Here's how the part is built. I have some questions about the finished solid (model axes, mm). Face numbers are marked on the shaded views. A direction names the side the tool comes from. Give positions to 0.01 mm unless a question says otherwise; leave off trailing zeros. Write each loop counter-clockwise with the first axis right and the second up, starting at its lowest first coordinate (ties: lowest second). Pieces come first, ordered by that corner, then holes. Notation, with made-up numbers: (59.5, 34.5) - (68.5, 34.5) arc R24 ccw to (68.5, 48.5) - close; hole circle Ø3 at (17, 10.5). An arc over 180 degrees is marked (long way). Write each question's results on one line, items separated by ' | '. Start each with the question number.
Item 1: Suppose I cut it at B-B on z = 0. List the corners of the cut face in (x, y) for me.
Item 2: Please list where these lines run through material, in increasing order: line 1 along X through (y, z) = (-3.75, 0); line 2 along Y through (x, z) = (14.5, 9.5); line 3 along Z through (x, y) = (-2.5, 0.75).
Item 3: Suppose I cut it at C-C on y = 1. List the corners of the cut face in (x, z) for me, then the cut area to 3 significant figures.
Item 4: We'd pull the mould along X, two halves only. Please class the marked faces 1, 2 and 3: +X half, -X half, draft (parallel to the pull), parting line (faces both ways), or undercut.
Item 5: Will these pins go through, and if not, where does the flat tip stop? P1, Ø1.5, axis at y = 5, z = 21, coming from the +X side; P2, Ø2, axis at x = -17, z = 15.5, coming from the -Y side; P3, Ø6, axis at y = 1, z = -18, coming from the +X side; P4, Ø8, axis at x = 0, z = 0, coming from the +Y side.
Item 6: Which directions (+Z, -Z, +X, -X, +Y, -Y) give clear straight access to the entire face, cutting with the end or side of a thin tool? Please do the marked faces 4 and 5.
Item 7: Suppose I cut it at A-A on x = 0. List the corners of the cut face in (y, z) for me.
```python
from build123d import *


with BuildPart() as part:
    # Sketch → Revolution (revolve)
    with BuildSketch(Plane.YZ):
        Polygon((7, 40), (-7, 40), (-4.57259, 33.620199), (-4.57259, 9.331906), (-7, 9.331906), (-7, 5), (7, 5), (7, 9.331906), (4.57259, 9.331906), (4.57259, 33.620199), align=None)
    revolve(axis=Axis((0, 0, 0), (0, 1, 0)))


solid = part.part
```
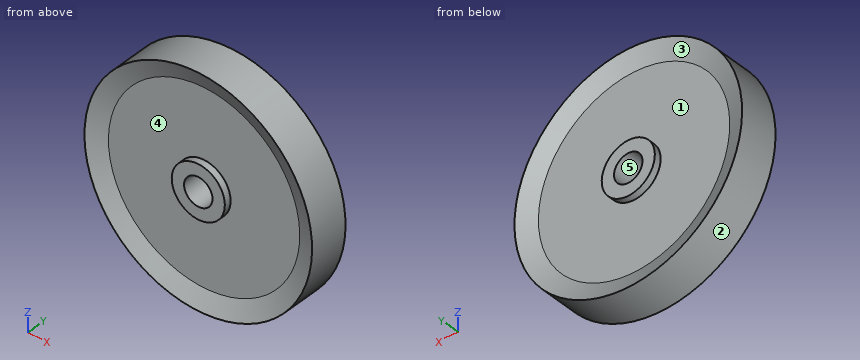
Checked values:
1) outline: (-40, -7) - (-33.62, -4.57) - (-9.33, -4.57) - (-9.33, -7) - (-5, -7) - (-5, 7) - (-9.33, 7) - (-9.33, 4.57) - (-33.62, 4.57) - (-40, 7) - close; (5, -7) - (9.33, -7) - (9.33, -4.57) - (33.62, -4.57) - (40, -7) - (40, 7) - (33.62, 4.57) - (9.33, 4.57) - (9.33, 7) - (5, 7) - close
2) line 1: x = -40 to -5, 5 to 40 | line 2: y = -4.57 to 4.57 | line 3: z = -39.92 to -4.33, 4.33 to 39.92
3) outline: circle Ø80 at (0, 0); hole circle Ø10 at (0, 0) | area: 4,950 mm^2
4) face 1: undercut | face 2: parting line | face 3: undercut
5) P1: stops at x = 34.5 | P2: stops at y = -4.57 | P3: stops at x = 37.08 | P4: passes through
6) face 4: -Y | face 5: +Y, -Y
7) outline: (-7, -40) - (7, -40) - (4.57, -33.62) - (4.57, -9.33) - (7, -9.33) - (7, -5) - (-7, -5) - (-7, -9.33) - (-4.57, -9.33) - (-4.57, -33.62) - close; (-7, 5) - (7, 5) - (7, 9.33) - (4.57, 9.33) - (4.57, 33.62) - (7, 40) - (-7, 40) - (-4.57, 33.62) - (-4.57, 9.33) - (-7, 9.33) - close
